Input: part model. Units: mm. Frame: model coordinates. Face numbers are marked on the shaded views. A direction names the side the tool comes from. Coordinates: 2 decimals unless noted, no trailing zeros. Order: outer loops, then holes, each group sorted by start corner. A loop starts at its lowest first (then second) coordinate and runs counter-clockwise, first axis right, second up.
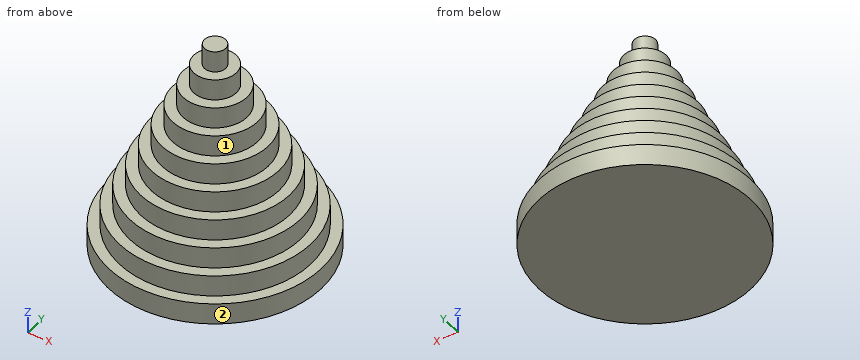
from build123d import *

# Parameters (mm, degrees)
F0_R      = 17.5
F0_R_2    = 15
F0_R_3    = 12.5
F0_R_4    = 10
F0_R_5    = 7.5
F0_R_6    = 5
F0_R_7    = 20
F0_R_8    = 25
F0_R_9    = 22.5
F0_R_10   = 2.5
F1_DEPTH  = 5
F2_DEPTH  = 10
F3_DEPTH  = 15
F4_DEPTH  = 20
F5_DEPTH  = 25
F6_DEPTH  = 30
F7_DEPTH  = 35
F8_DEPTH  = 40
F9_DEPTH  = 45
F10_DEPTH = 50


with BuildPart() as f1:
    # F0 (on Top) → F1 (new body)
    with BuildSketch(Plane.XY):
        Circle(F0_R)
        Circle(F0_R_2, mode=Mode.SUBTRACT)
        Circle(F0_R_3)
        Circle(F0_R_4, mode=Mode.SUBTRACT)
        Circle(F0_R_5)
        Circle(F0_R_6, mode=Mode.SUBTRACT)
        Circle(F0_R_4)
        Circle(F0_R_5, mode=Mode.SUBTRACT)
        Circle(F0_R_7)
        Circle(F0_R, mode=Mode.SUBTRACT)
        Circle(F0_R_2)
        Circle(F0_R_3, mode=Mode.SUBTRACT)
        Circle(F0_R_8)
        Circle(F0_R_9, mode=Mode.SUBTRACT)
        Circle(F0_R_10)
        Circle(F0_R_9)
        Circle(F0_R_7, mode=Mode.SUBTRACT)
        Circle(F0_R_6)
        Circle(F0_R_10, mode=Mode.SUBTRACT)
    extrude(amount=F1_DEPTH)

    # F0 (on Top) → F2 (join)
    with BuildSketch(Plane.XY):
        Circle(F0_R)
        Circle(F0_R_2, mode=Mode.SUBTRACT)
        Circle(F0_R_3)
        Circle(F0_R_4, mode=Mode.SUBTRACT)
        Circle(F0_R_5)
        Circle(F0_R_6, mode=Mode.SUBTRACT)
        Circle(F0_R_4)
        Circle(F0_R_5, mode=Mode.SUBTRACT)
        Circle(F0_R_7)
        Circle(F0_R, mode=Mode.SUBTRACT)
        Circle(F0_R_2)
        Circle(F0_R_3, mode=Mode.SUBTRACT)
        Circle(F0_R_10)
        Circle(F0_R_9)
        Circle(F0_R_7, mode=Mode.SUBTRACT)
        Circle(F0_R_6)
        Circle(F0_R_10, mode=Mode.SUBTRACT)
    extrude(amount=F2_DEPTH)

    # F0 (on Top) → F3 (join)
    with BuildSketch(Plane.XY):
        Circle(F0_R)
        Circle(F0_R_2, mode=Mode.SUBTRACT)
        Circle(F0_R_3)
        Circle(F0_R_4, mode=Mode.SUBTRACT)
        Circle(F0_R_5)
        Circle(F0_R_6, mode=Mode.SUBTRACT)
        Circle(F0_R_4)
        Circle(F0_R_5, mode=Mode.SUBTRACT)
        Circle(F0_R_7)
        Circle(F0_R, mode=Mode.SUBTRACT)
        Circle(F0_R_2)
        Circle(F0_R_3, mode=Mode.SUBTRACT)
        Circle(F0_R_10)
        Circle(F0_R_6)
        Circle(F0_R_10, mode=Mode.SUBTRACT)
    extrude(amount=F3_DEPTH)

    # F0 (on Top) → F4 (join)
    with BuildSketch(Plane.XY):
        Circle(F0_R_10)
        Circle(F0_R_6)
        Circle(F0_R_10, mode=Mode.SUBTRACT)
        Circle(F0_R_5)
        Circle(F0_R_6, mode=Mode.SUBTRACT)
        Circle(F0_R_4)
        Circle(F0_R_5, mode=Mode.SUBTRACT)
        Circle(F0_R_3)
        Circle(F0_R_4, mode=Mode.SUBTRACT)
        Circle(F0_R_2)
        Circle(F0_R_3, mode=Mode.SUBTRACT)
        Circle(F0_R)
        Circle(F0_R_2, mode=Mode.SUBTRACT)
    extrude(amount=F4_DEPTH)

    # F0 (on Top) → F5 (join)
    with BuildSketch(Plane.XY):
        Circle(F0_R_10)
        Circle(F0_R_6)
        Circle(F0_R_10, mode=Mode.SUBTRACT)
        Circle(F0_R_5)
        Circle(F0_R_6, mode=Mode.SUBTRACT)
        Circle(F0_R_4)
        Circle(F0_R_5, mode=Mode.SUBTRACT)
        Circle(F0_R_3)
        Circle(F0_R_4, mode=Mode.SUBTRACT)
        Circle(F0_R_2)
        Circle(F0_R_3, mode=Mode.SUBTRACT)
    extrude(amount=F5_DEPTH)

    # F0 (on Top) → F6 (join)
    with BuildSketch(Plane.XY):
        Circle(F0_R_10)
        Circle(F0_R_6)
        Circle(F0_R_10, mode=Mode.SUBTRACT)
        Circle(F0_R_5)
        Circle(F0_R_6, mode=Mode.SUBTRACT)
        Circle(F0_R_4)
        Circle(F0_R_5, mode=Mode.SUBTRACT)
        Circle(F0_R_3)
        Circle(F0_R_4, mode=Mode.SUBTRACT)
    extrude(amount=F6_DEPTH)

    # F0 (on Top) → F7 (join)
    with BuildSketch(Plane.XY):
        Circle(F0_R_4)
        Circle(F0_R_5, mode=Mode.SUBTRACT)
        Circle(F0_R_5)
        Circle(F0_R_6, mode=Mode.SUBTRACT)
        Circle(F0_R_6)
        Circle(F0_R_10, mode=Mode.SUBTRACT)
        Circle(F0_R_10)
    extrude(amount=F7_DEPTH)

    # F0 (on Top) → F8 (join)
    with BuildSketch(Plane.XY):
        Circle(F0_R_10)
        Circle(F0_R_6)
        Circle(F0_R_10, mode=Mode.SUBTRACT)
        Circle(F0_R_5)
        Circle(F0_R_6, mode=Mode.SUBTRACT)
    extrude(amount=F8_DEPTH)

    # F0 (on Top) → F9 (join)
    with BuildSketch(Plane.XY):
        Circle(F0_R_6)
        Circle(F0_R_10, mode=Mode.SUBTRACT)
        Circle(F0_R_10)
    extrude(amount=F9_DEPTH)

    # F0 (on Top) → F10 (join)
    with BuildSketch(Plane.XY):
        Circle(F0_R_10)
    extrude(amount=F10_DEPTH)


solid = f1.part
Item 1: Cut plane B-B on z = 36. Return loops of the section in (x, y).
Response values:
outline: circle Ø15 at (0, 0)
Item 2: Cut plane C-C on y = -14. Return loops of the section in (x, z).
Response values:
outline: (-20.71, 0) - (20.71, 0) - (20.71, 5) - (17.61, 5) - (17.61, 10) - (14.28, 10) - (14.28, 15) - (10.5, 15) - (10.5, 20) - (5.39, 20) - (5.39, 25) - (-5.39, 25) - (-5.39, 20) - (-10.5, 20) - (-10.5, 15) - (-14.28, 15) - (-14.28, 10) - (-17.61, 10) - (-17.61, 5) - (-20.71, 5) - close
Item 3: Access query for the marked faces 1 and 2. Directions: +Z, -Z, +X, -X, +Y, -Y. A direction counts if a zero-diameter tool reaches every point of the face in a straight line with its end or side. Return the directions, or none.
Response values:
face 1: +Z
face 2: +Z, -Z
Item 4: Pin query (flat end, axial travel): pin 1 Ø8 at (x, z) = (-7, 41.5) entering from -Y; pin 2 Ø10 at (y, z) = (-5.5, 39) entering from -X; pin 3 Ø1 at (x, z) = (-15.5, 14.5) entering from +Y. Return the tip coordinate at first contact, or that it passes through.
Response values:
pin 1: stops at y = -6.74
pin 2: stops at x = -9.68
pin 3: stops at y = 13.23
Item 5: Cut plane D-D on y = 11. Return loops of the section in (x, z), then the cut area to 3 significant figures.
Response values:
outline: (-22.45, 0) - (22.45, 0) - (22.45, 5) - (19.63, 5) - (19.63, 10) - (16.7, 10) - (16.7, 15) - (13.61, 15) - (13.61, 20) - (10.2, 20) - (10.2, 25) - (5.94, 25) - (5.94, 30) - (-5.94, 30) - (-5.94, 25) - (-10.2, 25) - (-10.2, 20) - (-13.61, 20) - (-13.61, 15) - (-16.7, 15) - (-16.7, 10) - (-19.63, 10) - (-19.63, 5) - (-22.45, 5) - close
area: 885 mm2
Item 6: Ray query, probe 1 along Z at (x, y) = (-1.5, 20); probe 2 along Z at (x, y) = (-9.5, -22); probe 3 along Y at (x, z) = (1.5, 10.5). Return the intervals inside material, ascending.
Response values:
probe 1: z = 0 to 10
probe 2: z = 0 to 5
probe 3: y = -19.94 to 19.94
Item 7: Cut plane A-A on x = 21.5. Return loops of the section in (y, z), then the cut area to 3 significant figures.
Response values:
outline: (-12.76, 0) - (12.76, 0) - (12.76, 5) - (6.63, 5) - (6.63, 10) - (-6.63, 10) - (-6.63, 5) - (-12.76, 5) - close
area: 194 mm2
